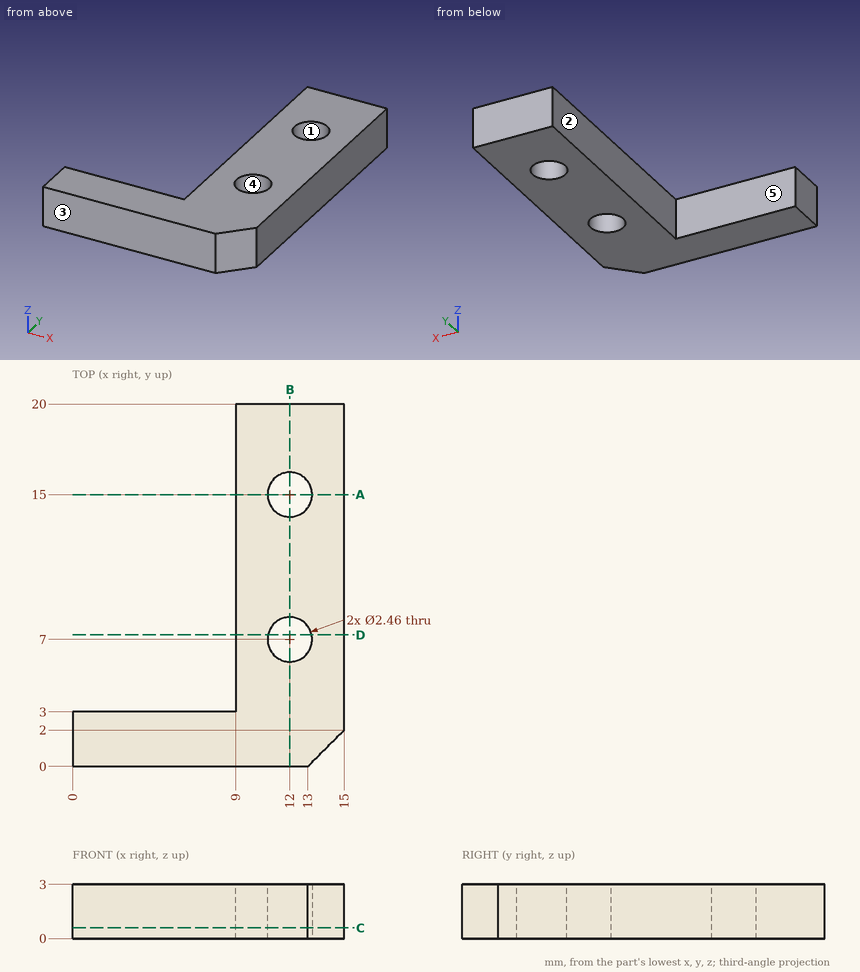
Design review of the part shown in the three views and the two pictorial views. Dimensions are in mm from the part's minimum x, y and z. A direction names the side the tool comes from. Round coordinates to 2 decimals unless told otherwise and drop trailing zeros. Write each loop counter-clockwise with the first axis right and the second up, starting at its lowest first coordinate (ties: lowest second). Pieces come first, ordered by that corner, then holes.
1) Mouldability with a two-part tool opening along Y and no side actions: class the marked faces 3, 4 and 5 as +Y half, -Y half, draft (parallel to the pull), parting line (faces both ways), or undercut.
Answer below:
face 3: -Y half
face 4: undercut
face 5: +Y half
2) Take a section at B-B on x = 12. Give the boundary of the cut face in (y, z), then the cut area to 3 significant figures.
Answer below:
outline: (0, 0) - (5.77, 0) - (5.77, 3) - (0, 3) - close; (8.23, 0) - (13.77, 0) - (13.77, 3) - (8.23, 3) - close; (16.23, 0) - (20, 0) - (20, 3) - (16.23, 3) - close
area: 45.2 mm2
3) Machinability: for the marked faces 1 and 2, which of the approach directions +Z, -Z, +X, -X, +Y, -Y give a long, thin tool a straight path to every point of the face, cutting with its end or side? Answer none if there is none.
Answer below:
face 1: +Z, -Z
face 2: +Z, -Z, -X, +Y
4) Take a section at D-D on y = 7.25. Give the boundary of the cut face in (x, z), then the cut area to 3 significant figures.
Answer below:
outline: (9, 0) - (10.8, 0) - (10.8, 3) - (9, 3) - close; (13.2, 0) - (15, 0) - (15, 3) - (13.2, 3) - close
area: 10.8 mm2
5) Insertion check: pin 1 Ø3 at (x, y) = (12, 15) entering from -Z; pin 2 Ø2 at (x, y) = (12, 7) entering from -Z; pin 3 Ø1 at (x, z) = (2, 2.5) entering from +Y; pin 4 Ø0.9 at (y, z) = (10, 1.5) entering from -X. Each pin has a flat end and moves straight along its axis. Give the tip position at first contact, or say it passes through.
Answer below:
pin 1: stops at z = 0
pin 2: passes through
pin 3: stops at y = 3
pin 4: stops at x = 9
6) Take a section at A-A on y = 15. Give the boundary of the cut face in (x, z), then the cut area to 3 significant figures.
Answer below:
outline: (9, 0) - (10.77, 0) - (10.77, 3) - (9, 3) - close; (13.23, 0) - (15, 0) - (15, 3) - (13.23, 3) - close
area: 10.6 mm2
7) Take a section at C-C on z = 0.6. Give the boundary of the cut face in (x, y).
Answer below:
outline: (0, 0) - (13, 0) - (15, 2) - (15, 20) - (9, 20) - (9, 3) - (0, 3) - close; hole circle Ø2.46 at (12, 7); hole circle Ø2.46 at (12, 15)
8) For line 1 along Y through (x, z) = (12, 2.05); line 2 along Y through (x, z) = (2.75, 1.1); line 3 along X through (y, z) = (10, 0.55), list the stretches that pass through material, from the lowest coordinate up.
Answer below:
line 1: y = 0 to 5.77, 8.23 to 13.77, 16.23 to 20
line 2: y = 0 to 3
line 3: x = 9 to 15
